For this review, take the finished solid that the model builds, in its own axes (mm). A direction names the side the tool comes from. Round coordinates to 2 decimals unless told otherwise and drop trailing zeros. Write each loop counter-clockwise with the first axis right and the second up, starting at its lowest first coordinate (ties: lowest second). Pieces come first, ordered by that corner, then holes. Notation, with made-up numbers: M 41,-2.5 L 47,-2.5 A29 ccw 47,33.5 Z; hole C 8.25,49.25 d2. An arc over 180 degrees is marked long. Use one line per item in the form item = value. Start each with the question number.
Item 1: Add section C-C (z = -1.5). State the section outline as (x, y) points.
Item 2: Draft analysis for pull direction Z (two halves, no side actions). For faces 1 (the flat face through (-4, 1, -2)), 2 (the flat face through (-1.2, 0.5, 1)), 3 (the cylindrical face through (-13.619, 0.493, -1.838)), state which applies: released by +Z, released by -Z, zero draft, split by the parting line, or undercut.
Item 3: Add section B-B (y = 0.7). State the section outline as (x, z) points.
Item 4: Add section D-D (x = -9.25). State the section outline as (y, z) points.
Item 5: Add section A-A (x = -13.25). State the section outline as (y, z) points.
Item 6: For line 1 (Z direction, x = -13.25, y = 0.45); line 2 (X direction, y = 0.6, z = -1.5); line 3 (X direction, y = 0.55, z = -3.3), list the stretches that pass through material, from the lowest coordinate up. Write a range as [from, to].
Item 7: For faces 4 (the flat face through (-1.3, 0.5, -4)), 5 (the flat face through (-9.8, 0.5, -3)), 6 (the flat face through (-9.7, 0.5, 0)), list the 3-axis set-ups (+Z, -Z, +X, -X, +Y, -Y) from which the entire face can be reached by the end or side of a thin tool; tool diameter is ignored.
from build123d import *

# Parameters (mm, degrees)
SKETCH1_R           = 0.5
BOSS_EXTRUDE1_DEPTH = 1
FILLET1_R           = 0.3


with BuildPart() as part:
    # Sketch1 → Boss-Extrude1 (new body)
    with BuildSketch(Plane(origin=(0, 0, 0), x_dir=(1, 0, 0), z_dir=(0, 1, 0))):
        Polygon((-4.5, 0), (-15, 0), (-15, 3), (-4.5, 3), (-4.5, 4), (2, 4), (2, -1), (-4.5, -1), align=None)
        with Locations((-13.25, 1.5)):
            Circle(SKETCH1_R, mode=Mode.SUBTRACT)
    extrude(amount=BOSS_EXTRUDE1_DEPTH)

    # Fillet1
    fillet1_edges = [part.edges().sort_by_distance(p)[0] for p in [
        (-15, 0.5, -3),
        (-4.5, 0.5, -3),
        (-4.5, 0.5, -4),
        (2, 0.5, -4),
        (2, 0.5, 1),
        (-4.5, 0.5, 1),
        (-4.5, 0.5, 0),
        (-15, 0.5, 0),
    ]]
    fillet(fillet1_edges, radius=FILLET1_R)


solid = part.part
Calculated:
q1.outline = M -15,0 L -13.75,0 L -13.75,1 L -15,1 Z; M -12.75,0 L 2,0 L 2,1 L -12.75,1 Z
q2.face_1 = zero draft
q2.face_2 = released by +Z
q2.face_3 = undercut
q3.outline = M -15,-2.7 A0.3 ccw -14.7,-3 L -4.8,-3 A0.3 cw -4.5,-3.3 L -4.5,-3.7 A0.3 ccw -4.2,-4 L 1.7,-4 A0.3 ccw 2,-3.7 L 2,0.7 A0.3 ccw 1.7,1 L -4.2,1 A0.3 ccw -4.5,0.7 L -4.5,0.3 A0.3 cw -4.8,0 L -14.7,0 A0.3 ccw -15,-0.3 Z; hole C -13.25,-1.5 d1
q4.outline = M 0,-3 L 1,-3 L 1,0 L 0,0 Z
q5.outline = M 0,-3 L 1,-3 L 1,-2 L 0,-2 Z; M 0,-1 L 1,-1 L 1,0 L 0,0 Z
q6.line_1 = [-3, -2], [-1, 0]
q6.line_2 = [-15, -13.75], [-12.75, 2]
q6.line_3 = [-4.5, 2]
q7.face_4 = -Z, +X, -X, +Y, -Y
q7.face_5 = -Z, -X, +Y, -Y
q7.face_6 = +Z, -X, +Y, -Y
